```python
from build123d import *

# Parameters (mm, degrees)
BOSS_EXTRUDE1_DEPTH = 17.5
SKETCH2_R           = 6
CUT_EXTRUDE1_DEPTH  = 35
SKETCH3_R           = 2
FILLET1_DEPTH       = 35
FILLET2_DEPTH       = 35
CUT_EXTRUDE2_START  = -8
SKETCH4_R           = 10
CUT_EXTRUDE2_DEPTH  = 35


with BuildPart() as part:
    # Sketch1 → Boss-Extrude1 (new, symmetric)
    with BuildSketch(Plane(origin=(0, 0, 0), x_dir=(1, 0, 0), z_dir=(0, 1, 0))):
        with BuildLine():
            Line((30, 0), (65, 0))
            Line((65, 0), (65, -10))
            Line((65, -10), (53.619026474, -10))
            ThreePointArc((53.619026474, -10), (38.828827016, -13.278556149), (26.809513237, -22.5))
            ThreePointArc((26.809513237, -22.5), (0, -35), (-26.809513237, -22.5))
            ThreePointArc((-26.809513237, -22.5), (-38.828827016, -13.278556149), (-53.619026474, -10))
            Line((-53.619026474, -10), (-65, -10))
            Line((-65, -10), (-65, 0))
            Line((-65, 0), (-30, 0))
            ThreePointArc((-30, 0), (0, -30), (30, 0))
        make_face()
    extrude(amount=BOSS_EXTRUDE1_DEPTH, both=True)

    # Sketch2 → Cut-Extrude1 (cut)
    with BuildSketch(Plane(origin=(0, 0, 0), x_dir=(-1, 0, 0), z_dir=(0, 0, -1))):
        with Locations((47.5, 0)):
            Circle(SKETCH2_R)
        with Locations((-47.5, 0)):
            Circle(SKETCH2_R)
    extrude(amount=-CUT_EXTRUDE1_DEPTH, mode=Mode.SUBTRACT)

    # Sketch3 → Cut-Revolve1 (revolve, cut)
    with BuildSketch(Plane(origin=(0, 0, 0), x_dir=(-1, 0, 0), z_dir=(0, 0, -1))):
        with Locations((30, 0)):
            Circle(SKETCH3_R)
    revolve(axis=Axis((0, 17.5, 0), (0, -1, 0)), mode=Mode.SUBTRACT)

    # Fillet1: read off the stored shape, not the designer's step
    # Fillet1 outline → Fillet1 (cut)
    with BuildSketch(Plane.XY):
        with BuildLine():
            Line((65, 17.5), (47.5, 17.5))
            ThreePointArc((47.5, 17.5), (59.87436864, 12.374368701), (65, 8.6e-08))
            Line((65, 8.6e-08), (65, 17.5))
        make_face()
        with BuildLine():
            Line((65, -17.5), (65, 8.6e-08))
            ThreePointArc((65, 8.6e-08), (59.874368701, -12.374368641), (47.499999999, -17.5))
            Line((47.499999999, -17.5), (65, -17.5))
        make_face()
    extrude(amount=FILLET1_DEPTH, mode=Mode.SUBTRACT)

    # Fillet2: read off the stored shape, not the designer's step
    # Fillet2 outline → Fillet2 (cut)
    with BuildSketch(Plane.XY):
        with BuildLine():
            ThreePointArc((-47.5, -17.5), (-59.874368677, -12.374368665), (-65, 1.8e-08))
            Line((-65, 1.8e-08), (-65, -17.5))
            Line((-65, -17.5), (-47.5, -17.5))
        make_face()
        with BuildLine():
            ThreePointArc((-65, 1.8e-08), (-59.874368665, 12.374368677), (-47.5, 17.5))
            Line((-47.5, 17.5), (-65, 17.5))
            Line((-65, 17.5), (-65, 1.8e-08))
        make_face()
    extrude(amount=FILLET2_DEPTH, mode=Mode.SUBTRACT)

    # Sketch4 → Cut-Extrude2 (cut)
    with BuildSketch(Plane(origin=(0, 0, 0), x_dir=(-1, 0, 0), z_dir=(0, 0, -1)).offset(CUT_EXTRUDE2_START)):
        with Locations((-47.5, 0)):
            Circle(SKETCH4_R)
        with Locations((47.5, 0)):
            Circle(SKETCH4_R)
    extrude(amount=-CUT_EXTRUDE2_DEPTH, mode=Mode.SUBTRACT)


solid = part.part
```
Part model, mm, in its own coordinate system. A direction names the side the tool comes from. Round coordinates to 2 decimals unless told otherwise and drop trailing zeros. Loops run counter-clockwise (first coordinate to the right, second up) from the corner with the lowest first, then second, coordinate; pieces in that order, holes last. Notation, with made-up numbers: (76.5, 65.25) -> (110.5, 65.25) arc R21 cw to (110.5, 100.25) -> close; hole circle Ø6 at (80.25, 9). An arc over 180 degrees is marked (long way). Use one line per item in the form item = value. Start each with the question number.
Item 1: Drill centre lines: line 1 along Y through (x, z) = (-47.5, 5.25); line 2 along X through (y, z) = (3, 2); line 3 along Y through (x, z) = (-47, 9). Where is each one in solid material? Low to high.
Item 2: Drop flat-ended pins along their axis: pin 1 Ø4 at (x, y) = (-14.5, -6.5) entering from -Z; pin 2 Ø12 at (x, z) = (36.5, 14.5) entering from +Y; pin 3 Ø8 at (x, y) = (-0.5, 13) entering from +Z; pin 4 Ø16 at (x, y) = (-42.5, -2) entering from +Z. Give the stop position or say it passes through.
Item 3: Tool access for faces 4 (the cylindrical face through (-0.66, -9.642, 29.993)), 5 (the flat face through (-47, -7, 8)), 6 (the flat face through (-59, 0, 10)), 7 (the flat face through (59, 0, 10)): list every direction of +Z, -Z, +X, -X, +Y, -Y with a clear straight run to the whole face (end or side of a thin tool).
Item 4: Band-saw the part on A-A (y = 11.5). List the corners of the cut face in (x, z), plus the area to 3 significant figures.
Item 5: Band-saw the part on B-B (x = 0). List the corners of the cut face in (y, z), plus the area to 3 significant figures.
Item 6: Band-saw the part on C-C (x = 39.5). List the corners of the cut face in (y, z), plus the area to 3 significant figures.
Item 7: Two-plate mould, pull along Y, no slides. Class faces 1 (the cylindrical face through (-0.66, 9.858, 29.993)), 2 (the flat face through (0, 17.5, 32)), 3 (the cylindrical face through (37.96, 3, 9.61)): released by +Y, released by -Y, zero draft, split by the parting line, or undercut.
Data:
q1.line_1 = -17.5 to -6, 6 to 17.5
q1.line_2 = -64.74 to -52.7, -42.3 to -29.93, 29.93 to 42.3, 52.7 to 64.74
q1.line_3 = -17.5 to -9.99, 9.99 to 17.5
q2.pin_1 = 25.05
q2.pin_2 = 17.5
q2.pin_3 = 35
q2.pin_4 = 15.68
q3.face_4 = -Z, +Y, -Y
q3.face_5 = +Z
q3.face_6 = +Z, -X, +Y, -Y
q3.face_7 = +Z, +X, +Y, -Y
q4.outline = (-60.69, 0) -> (-30, 0) arc R30 cw to (30, 0) -> (60.69, 0) -> (60.69, 10) -> (53.62, 10) arc R35 cw to (26.81, 22.5) arc R35 ccw to (-26.81, 22.5) arc R35 cw to (-53.62, 10) -> (-60.69, 10) -> close
q4.area = 1,140 mm^2
q5.outline = (-17.5, 30) -> (-2, 30) arc R2 cw to (2, 30) -> (17.5, 30) -> (17.5, 35) -> (-17.5, 35) -> close
q5.area = 169 mm^2
q6.outline = (-17.5, 0) -> (17.5, 0) -> (17.5, 12.97) -> (6, 12.97) -> (6, 8) -> (-6, 8) -> (-6, 12.97) -> (-17.5, 12.97) -> close
q6.area = 394 mm^2
q7.face_1 = zero draft
q7.face_2 = released by +Y
q7.face_3 = undercut
